Can you work these out from the model? Positions are in its coordinate system, mm. Give positions to 0.01 mm unless a question says otherwise; leave off trailing zeros. Loops run counter-clockwise (first coordinate to the right, second up) from the corner with the lowest first, then second, coordinate; pieces in that order, holes last. Notation, with made-up numbers: (64.5, 47) - (91.5, 47) arc R16 ccw to (91.5, 77) - close; hole circle Ø7 at (-3.75, 87.5). An arc over 180 degrees is marked (long way). Answer as a JSON object with one key per item and string values. Group by question number.
Item 1: Will these pins go through, and if not, where does the flat tip stop? pin 1 (1.2 mm diameter, centred on y = -50, z = 1, fed in from +X); pin 2 (3.5 mm diameter, centred on x = 19.47, y = -57, fed in from +Z); pin 3 (2 mm diameter, centred on y = -6, z = 0.5, fed in from -X); pin 4 (2 mm diameter, centred on y = -60, z = 2, fed in from -X).
Item 2: Please list where these lines run through material, in increasing order: L1, parallel to Y at x = -53.5, z = 2.25; L2, parallel to Y at x = 19, z = 2.65; L3, parallel to X at y = 2, z = 0.9 (3 decimals).
Item 3: Suppose I cut it at A-A on y = 8. Write out the boundary of the cut face in (x, z).
Item 4: Suppose I cut it at D-D on x = -20. Write out the boundary of the cut face in (y, z).
Item 5: Suppose I cut it at C-C on y = -18. Write out the boundary of the cut face in (x, z).
Item 6: Suppose I cut it at B-B on x = -44.5. Write out the boundary of the cut face in (y, z).
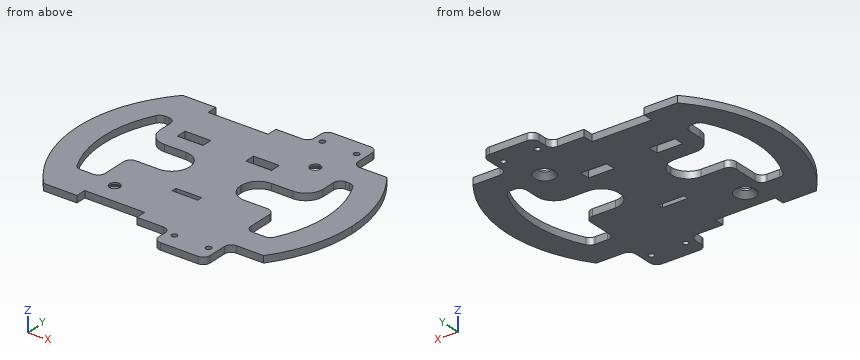
from build123d import *

# Parameters (mm, degrees)
ESBO_O1_R                = 3.05
ESBO_O1_W                = 15
ESBO_O1_H                = 3
ESBO_O1_R_2              = 1.6
ESBO_O1_H_2              = 6
RESSALTO_EXTRUS_O1_DEPTH = 4
CHANFRO1_SIZE            = 3
FILETE1_R                = 4
FILETE2_R                = 10


with BuildPart() as part:
    # Esboço1 → Ressalto-extrusão1 (new body)
    with BuildSketch(Plane.XY):
        with BuildLine():
            Line((14.471901241, -53.5), (14.471901241, -66.5))
            Line((14.471901241, -66.5), (44.471901241, -66.5))
            Line((44.471901241, -66.5), (44.471901241, -47.5))
            Line((44.471901241, -47.5), (64.371965948, -47.5))
            ThreePointArc((64.371965948, -47.5), (75.99262226, -25.002427124), (80, 0))
            ThreePointArc((80, 0), (75.99262226, 25.002427124), (64.371965948, 47.5))
            Line((64.371965948, 47.5), (44.471901241, 47.5))
            Line((44.471901241, 47.5), (44.471901241, 66.5))
            Line((44.471901241, 66.5), (14.471901241, 66.5))
            Line((14.471901241, 66.5), (14.471901241, 53.5))
            Line((14.471901241, 53.5), (-5.003543323, 53.5))
            Line((-5.003543323, 53.5), (-5.003543323, 47.5))
            Line((-5.003543323, 47.5), (-40.003543323, 47.5))
            Line((-40.003543323, 47.5), (-40.003543323, 53.5))
            Line((-40.003543323, 53.5), (-59.478987886, 53.5))
            ThreePointArc((-59.478987886, 53.5), (-74.693771597, 28.650313865), (-80, 0))
            ThreePointArc((-80, 0), (-74.693771597, -28.650313865), (-59.478987886, -53.5))
            Line((-59.478987886, -53.5), (-40.003543323, -53.5))
            Line((-40.003543323, -53.5), (-40.003543323, -47.5))
            Line((-40.003543323, -47.5), (-5.003543323, -47.5))
            Line((-5.003543323, -47.5), (-5.003543323, -53.5))
            Line((-5.003543323, -53.5), (14.471901241, -53.5))
        make_face()
        with BuildLine():
            ThreePointArc((-56.291651246, -32.5), (-65, 0), (-56.291651246, 32.5))
            Line((-56.291651246, 32.5), (-47.55, 32.5))
            Line((-47.55, 32.5), (-47.55, 10.5))
            Line((-47.55, 10.5), (-15, 10.5))
            Line((-15, 10.5), (-15, -10.2))
            Line((-15, -10.2), (-42.5, -10.2))
            Line((-42.5, -10.2), (-42.5, -32.5))
            Line((-42.5, -32.5), (-56.291651246, -32.5))
        make_face(mode=Mode.SUBTRACT)
        with Locations((-31.783703802, -35.29937921)):
            Circle(ESBO_O1_R, mode=Mode.SUBTRACT)
        with Locations((0, -21.7)):
            Rectangle(ESBO_O1_W, ESBO_O1_H, mode=Mode.SUBTRACT)
        with Locations((19.471901241, -57)):
            Circle(ESBO_O1_R_2, mode=Mode.SUBTRACT)
        with Locations((39.471901241, -57)):
            Circle(ESBO_O1_R_2, mode=Mode.SUBTRACT)
        with BuildLine():
            Line((42.5, -10.2), (15, -10.2))
            Line((15, -10.2), (15, 10.5))
            Line((15, 10.5), (47.55, 10.5))
            Line((47.55, 10.5), (47.55, 32.5))
            Line((47.55, 32.5), (56.291651246, 32.5))
            ThreePointArc((56.291651246, 32.5), (65, 0), (56.291651246, -32.5))
            Line((56.291651246, -32.5), (42.5, -32.5))
            Line((42.5, -32.5), (42.5, -10.2))
        make_face(mode=Mode.SUBTRACT)
        with Locations((-30.05, 23.5)):
            Rectangle(ESBO_O1_W, ESBO_O1_H_2, mode=Mode.SUBTRACT)
        with Locations((9.95, 23.5)):
            Rectangle(ESBO_O1_W, ESBO_O1_H_2, mode=Mode.SUBTRACT)
        with Locations((31.783703802, 35.29937921)):
            Circle(ESBO_O1_R, mode=Mode.SUBTRACT)
        with Locations((19.471901241, 57)):
            Circle(ESBO_O1_R_2, mode=Mode.SUBTRACT)
        with Locations((39.471901241, 57)):
            Circle(ESBO_O1_R_2, mode=Mode.SUBTRACT)
    extrude(amount=RESSALTO_EXTRUS_O1_DEPTH)

    # Chanfro1
    chanfro1_edges = [part.edges().sort_by_distance(p)[0] for p in [
        (-34.833703802, -35.29937921, 0),
        (28.733703802, 35.29937921, 0),
    ]]
    chamfer(chanfro1_edges, length=CHANFRO1_SIZE)

    # Filete1
    filete1_edges = [part.edges().sort_by_distance(p)[0] for p in [
        (56.291651246, 32.5, 2),
        (47.55, 32.5, 2),
        (42.5, -10.2, 2),
        (42.5, -32.5, 2),
        (56.291651246, -32.5, 2),
        (14.471901241, 53.5, 2),
        (14.471901241, 66.5, 2),
        (44.471901241, 66.5, 2),
        (44.471901241, 47.5, 2),
        (44.471901241, -47.5, 2),
        (44.471901241, -66.5, 2),
        (14.471901241, -66.5, 2),
        (14.471901241, -53.5, 2),
        (-42.5, -32.5, 2),
        (-42.5, -10.2, 2),
        (-47.55, 32.5, 2),
        (-56.291651246, 32.5, 2),
        (-56.291651246, -32.5, 2),
    ]]
    fillet(filete1_edges, radius=FILETE1_R)

    # Filete2
    filete2_edges = [part.edges().sort_by_distance(p)[0] for p in [
        (47.55, 10.5, 2),
        (15, 10.5, 2),
        (15, -10.2, 2),
        (-15, -10.2, 2),
        (-15, 10.5, 2),
        (-47.55, 10.5, 2),
    ]]
    fillet(filete2_edges, radius=FILETE2_R)


solid = part.part
Worked out:
{
 "1": {"pin 1": "stops at x = 45.07", "pin 2": "stops at z = 4", "pin 3": "stops at x = -79.84", "pin 4": "stops at x = 14.47"},
 "2": {"L1": "y = -53.5 to -32.5, 32.5 to 53.5", "L2": "y = -66.5 to -58.53, -55.47 to -8.2, 8.5 to 55.47, 58.53 to 66.5", "L3": "x = -79.975 to -64.969, -15.113 to 15.113, 64.969 to 79.975"},
 "3": {"outline": "(-79.6, 0) - (-64.51, 0) - (-64.51, 4) - (-79.6, 4) - close; (-18.39, 0) - (18.39, 0) - (18.39, 4) - (-18.39, 4) - close; (64.51, 0) - (79.6, 0) - (79.6, 4) - (64.51, 4) - close"},
 "4": {"outline": "(-47.5, 0) - (-8.86, 0) - (-8.86, 4) - (-47.5, 4) - close; (9.16, 0) - (47.5, 0) - (47.5, 4) - (9.16, 4) - close"},
 "5": {"outline": "(-77.95, 0) - (-62.46, 0) - (-62.46, 4) - (-77.95, 4) - close; (-42.5, 0) - (42.5, 0) - (42.5, 4) - (-42.5, 4) - close; (62.46, 0) - (77.95, 0) - (77.95, 4) - (62.46, 4) - close"},
 "6": {"outline": "(-53.5, 0) - (-31.96, 0) - (-31.96, 4) - (-53.5, 4) - close; (13.31, 0) - (53.5, 0) - (53.5, 4) - (13.31, 4) - close"}
}
